The model under review builds one solid part; all positions refer to its coordinate system, in mm. Coordinates: 2 decimals unless noted, no trailing zeros. Order: outer loops, then holes, each group sorted by start corner. A loop starts at its lowest first (then second) coordinate and runs counter-clockwise, first axis right, second up.
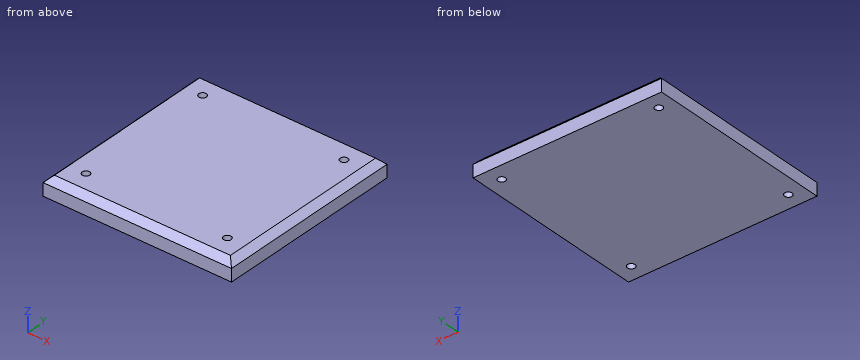
from build123d import *

# Parameters (mm, degrees)
F0_W          = 300
F0_H          = 300
F0_R          = 6
F1_DEPTH      = 15
F2_SIZE2      = 10
F2_SIZE       = 10
F3_DEPTH      = 5
F3_DEPTH_BACK = 15
F4_DEPTH      = 5
F4_DEPTH_BACK = 15


with BuildPart() as f1:
    # F0 (on Top) → F1 (new body, symmetric)
    with BuildSketch(Plane.XY):
        Rectangle(F0_W, F0_H)
        with Locations((-125, -125)):
            Circle(F0_R, mode=Mode.SUBTRACT)
        with Locations((-112.5, -112.5)):
            Circle(F0_R, mode=Mode.SUBTRACT)
        with Locations((125, -125)):
            Circle(F0_R, mode=Mode.SUBTRACT)
        with Locations((112.5, -112.5)):
            Circle(F0_R, mode=Mode.SUBTRACT)
        with Locations((-125, 125)):
            Circle(F0_R, mode=Mode.SUBTRACT)
        with Locations((-112.5, 112.5)):
            Circle(F0_R, mode=Mode.SUBTRACT)
        with Locations((112.5, 112.5)):
            Circle(F0_R, mode=Mode.SUBTRACT)
        with Locations((125, 125)):
            Circle(F0_R, mode=Mode.SUBTRACT)
    extrude(amount=F1_DEPTH, both=True)

    # F2
    f2_edges = [f1.edges().sort_by_distance(p)[0] for p in [
        (0, 150, 15),
        (0, -150, 15),
        (150, 0, 15),
        (-150, 0, 15),
    ]]
    chamfer(f2_edges, length=F2_SIZE, length2=F2_SIZE2)

    # F0 (on Top) → F3 (join, two sides)
    with BuildSketch(Plane.XY) as f3_sk:
        with Locations((-112.5, 112.5)):
            Circle(F0_R)
        with Locations((112.5, 112.5)):
            Circle(F0_R)
        with Locations((112.5, -112.5)):
            Circle(F0_R)
        with Locations((-112.5, -112.5)):
            Circle(F0_R)
    extrude(amount=F3_DEPTH)
    extrude(f3_sk.sketch, amount=-F3_DEPTH_BACK)

    # F0 (on Top) → F4 (join, two sides)
    with BuildSketch(Plane.XY) as f4_sk:
        with Locations((-125, 125)):
            Circle(F0_R)
        with Locations((125, 125)):
            Circle(F0_R)
        with Locations((125, -125)):
            Circle(F0_R)
        with Locations((-125, -125)):
            Circle(F0_R)
    extrude(amount=-F4_DEPTH)
    extrude(f4_sk.sketch, amount=F4_DEPTH_BACK)


solid = f1.part
(1) Insertion check: pin 1 Ø6 at (x, z) = (-94.5, 11.5) entering from -Y; pin 2 Ø3 at (y, z) = (-67.5, 7.5) entering from +X; pin 3 Ø15.5 at (x, y) = (112.5, 112.5) entering from +Z; pin 4 Ø3.5 at (x, y) = (-124, -125.5) entering from -Z. Each pin has a flat end and moves straight along its axis. Give the tip position at first contact, or say it passes through.
(2) Consider section A-A (y = 112.5). Give the boundary of the cut face in (x, z), then the cut area to 3 significant figures.
(3) Consider section B-B (x = 125). Give the boundary of the cut face in (y, z), then the cut area to 3 significant figures.
(4) Wall thickness on line 1 (Y direction, x = -125, z = -11.5); line 2 (X direction, y = -122, z = -11.75); line 3 (X direction, y = -127.5, z = 13.25): over which ranges is each line inside the solid? List them lowest first.
Findings:
1. pin 1: stops at y = -146.5
1. pin 2: stops at x = 149
1. pin 3: stops at z = 15
1. pin 4: stops at z = -5
2. outline: (-150, -15) - (150, -15) - (150, 5) - (140, 15) - (118.5, 15) - (118.5, 5) - (106.5, 5) - (106.5, 15) - (-106.5, 15) - (-106.5, 5) - (-118.5, 5) - (-118.5, 15) - (-140, 15) - (-150, 5) - close
2. area: 8,660 mm2
3. outline: (-150, -15) - (-131, -15) - (-131, -5) - (-119, -5) - (-119, -15) - (119, -15) - (119, -5) - (131, -5) - (131, -15) - (150, -15) - (150, 5) - (140, 15) - (-140, 15) - (-150, 5) - close
3. area: 8,660 mm2
4. line 1: y = -150 to -131, -119 to 119, 131 to 150
4. line 2: x = -150 to -130.2, -119.8 to 119.8, 130.2 to 150
4. line 3: x = -141.75 to 141.75
